```python
from build123d import *

# Parameters (mm, degrees)
SKETCH1_R               = 25
BOSS_EXTRUDE1_DEPTH     = 144
DOME1_FACE_RADIUS       = 25
DOME1_HEIGHT            = 15
DOME2_FACE_RADIUS       = 25
DOME2_HEIGHT            = 15
CUT_EXTRUDE3_DEPTH      = 2
CUT_EXTRUDE3_DEPTH_BACK = 20
SKETCH3_W               = 3
SKETCH3_H               = 25.725601723
SKETCH3_W_2             = 25.013024677
SKETCH3_H_2             = 3
CUT_EXTRUDE4_DEPTH      = 30


with BuildPart() as part:
    # Sketch1 → Boss-Extrude1 (new body)
    with BuildSketch(Plane.XY):
        Circle(SKETCH1_R)
    extrude(amount=BOSS_EXTRUDE1_DEPTH)

    # Dome1: a dome of height H over a round flat face of radius A is a cap of a sphere of radius (A * A + H * H) / (2 * H)
    dome1_r = (DOME1_FACE_RADIUS * DOME1_FACE_RADIUS + DOME1_HEIGHT * DOME1_HEIGHT) / (2 * DOME1_HEIGHT)
    dome1_base = Plane((0, 0, 144), z_dir=(0, 0, 1))
    with Locations(dome1_base.offset(DOME1_HEIGHT - dome1_r)):
        dome1_ball = Sphere(dome1_r, mode=Mode.PRIVATE)
    add(split(dome1_ball, bisect_by=dome1_base, keep=Keep.TOP, mode=Mode.PRIVATE))

    # Dome2: a dome of height H over a round flat face of radius A is a cap of a sphere of radius (A * A + H * H) / (2 * H)
    dome2_r = (DOME2_FACE_RADIUS * DOME2_FACE_RADIUS + DOME2_HEIGHT * DOME2_HEIGHT) / (2 * DOME2_HEIGHT)
    dome2_base = Plane((0, 0, 0), z_dir=(0, 0, -1))
    with Locations(dome2_base.offset(DOME2_HEIGHT - dome2_r)):
        dome2_ball = Sphere(dome2_r, mode=Mode.PRIVATE)
    add(split(dome2_ball, bisect_by=dome2_base, keep=Keep.TOP, mode=Mode.PRIVATE))

    # Sketch2 → Cut-Extrude3 (cut, two sides)
    with BuildSketch(Plane.XY) as cut_extrude3_sk:
        with BuildLine():
            Line((-1.5, 24.954959427), (-1.5, 1.5))
            Line((-1.5, 1.5), (-24.954959427, 1.5))
            ThreePointArc((-24.954959427, 1.5), (-25, 0), (-24.954959427, -1.5))
            Line((-24.954959427, -1.5), (-1.5, -1.5))
            Line((-1.5, -1.5), (-1.5, -24.954959427))
            ThreePointArc((-1.5, -24.954959427), (0, -25), (1.5, -24.954959427))
            Line((1.5, -24.954959427), (1.5, -1.5))
            Line((1.5, -1.5), (24.954959427, -1.5))
            ThreePointArc((24.954959427, -1.5), (24.98873732, -0.750338033), (25, 0))
            ThreePointArc((25, 0), (24.98873732, 0.750338033), (24.954959427, 1.5))
            Line((24.954959427, 1.5), (1.5, 1.5))
            Line((1.5, 1.5), (1.5, 24.954959427))
            ThreePointArc((1.5, 24.954959427), (0, 25), (-1.5, 24.954959427))
        make_face()
    extrude(amount=CUT_EXTRUDE3_DEPTH, mode=Mode.SUBTRACT)
    extrude(cut_extrude3_sk.sketch, amount=-CUT_EXTRUDE3_DEPTH_BACK, mode=Mode.SUBTRACT)

    # Sketch3 → Cut-Extrude4 (cut)
    with BuildSketch(Plane.XY.offset(170)):
        with Locations((0, -14.362800862)):
            Rectangle(SKETCH3_W, SKETCH3_H)
        with Locations((0, 14.362800862)):
            Rectangle(SKETCH3_W, SKETCH3_H)
        with Locations((14.006512339, 0)):
            Rectangle(SKETCH3_W_2, SKETCH3_H_2)
        with Locations((-14.006512339, 0)):
            Rectangle(SKETCH3_W_2, SKETCH3_H_2)
        Rectangle(SKETCH3_W, SKETCH3_H_2)
    extrude(amount=-CUT_EXTRUDE4_DEPTH, mode=Mode.SUBTRACT)


solid = part.part
```
The model under review builds one solid part; all positions refer to its coordinate system, in mm. A direction names the side the tool comes from. Round coordinates to 2 decimals unless told otherwise and drop trailing zeros. Order: outer loops, then holes, each group sorted by start corner. A loop starts at its lowest first (then second) coordinate and runs counter-clockwise, first axis right, second up. Notation, with made-up numbers: (82, -20.75) - (138, -20.75) arc R26 ccw to (138, -1.75) - close; hole circle Ø7 at (-23, -31). An arc over 180 degrees is marked (long way). Answer in a Markdown table with one row per item.
(1) Clearance check with flat-ended pins moving along their axes: P1, Ø5, axis at y = -12.5, z = -6, coming from the -X side; P2, Ø15, axis at x = 18, z = 151, coming from the +Y side; P3, Ø13.5, axis at y = 12, z = -3, coming from the -X side; P4, Ø8, axis at y = 1, z = 109.5, coming from the -X side. State where each tip first meets the part, or that it passes through.
Result set:
| item | result |
|---|---|
| P1 | stops at x = -19.53 |
| P2 | stops at y = 20.41 |
| P3 | stops at x = -24.28 |
| P4 | stops at x = -25 |
(2) Take a section at C-C on z = 31. Write out the cut boundary in (x, y).
Result set:
| item | result |
|---|---|
| outline | circle Ø50 at (0, 0) |
(3) Take a section at A-A on y = -11.5. Write out the cut boundary in (x, z).
Result set:
| item | result |
|---|---|
| outline | (-22.2, 0) arc R25.89 ccw to (-1.5, -12.52) - (-1.5, 2) - (1.5, 2) - (1.5, -12.52) arc R25.89 ccw to (22.2, 0) - (22.2, 144) arc R25.89 ccw to (1.5, 156.52) - (1.5, 140) - (-1.5, 140) - (-1.5, 156.52) arc R25.89 ccw to (-22.2, 144) - close |
(4) Machinability: for faces 1 (the face through (-11, 1.5, 147)), 2 (the face through (11, 1.5, -5)), 3 (the face through (-1.5, -10, -4)), 4 (the face through (0, 0, 2)), which of the approach directions +Z, -Z, +X, -X, +Y, -Y give a long, thin tool a straight path to every point of the face, cutting with its end or side? Answer none if there is none.
Result set:
| item | result |
|---|---|
| face 1 | +Z, +X, -X |
| face 2 | -Z, +X, -X |
| face 3 | -Z, +Y, -Y |
| face 4 | -Z |
(5) Mouldability with a two-part tool opening along X and no side actions: class faces 5 (the face through (10, 1.5, 147)), 6 (the face through (23.846, 7.509, 70.992)), 7 (the face through (1.5, -11, -5)) as released by +X, released by -X, zero draft, split by the parting line, or undercut.
Result set:
| item | result |
|---|---|
| face 5 | zero draft |
| face 6 | split by the parting line |
| face 7 | undercut |
(6) Take a section at B-B on x = 10.5. Write out the cut boundary in (y, z).
Result set:
| item | result |
|---|---|
| outline | (-22.69, 0) arc R26.32 ccw to (-1.5, -12.94) - (-1.5, 2) - (1.5, 2) - (1.5, -12.94) arc R26.32 ccw to (22.69, 0) - (22.69, 144) arc R26.32 ccw to (1.5, 156.94) - (1.5, 140) - (-1.5, 140) - (-1.5, 156.94) arc R26.32 ccw to (-22.69, 144) - close |
(7) For line 1 (Z direction, x = 0, y = 16); line 2 (X direction, y = 1, z = 31); line 3 (Y direction, x = 0, z = 32.5), list the stretches that pass through material, from the lowest coordinate up. Write a range as from..to.
Result set:
| item | result |
|---|---|
| line 1 | z = 2..140 |
| line 2 | x = -24.98..24.98 |
| line 3 | y = -25..25 |
